```python
from build123d import *

# Parameters (mm, degrees)
F1_DEPTH = 70
F2_R     = 5
F3_R     = 2


with BuildPart() as f1:
    # F0 (on Front) → F1 (new body)
    with BuildSketch(Plane.XZ):
        Polygon((14.728606, 17.047576), (0, 17.047576), (-14.728606, 17.047576), (-5.480258, -11.053172), (0, -11.053172), (5.480258, -11.053172), align=None)
        Polygon((-7.819207, 12.047576), (0, 12.047576), (7.819207, 12.047576), (1.861998, -6.053172), (0, -6.053172), (-1.861998, -6.053172), align=None, mode=Mode.SUBTRACT)
    extrude(amount=F1_DEPTH)

    # F2
    f2_edges = [f1.edges().sort_by_distance(p)[0] for p in [
        (14.728606, -35, 17.047576),
        (5.480258, -35, -11.053172),
        (-5.480258, -35, -11.053172),
        (-14.728606, -35, 17.047576),
    ]]
    fillet(f2_edges, radius=F2_R)

    # F3
    f3_edges = [f1.edges().sort_by_distance(p)[0] for p in [
        (-1.861998, -35, -6.053172),
        (1.861998, -35, -6.053172),
        (7.819207, -35, 12.047576),
        (-7.819207, -35, 12.047576),
    ]]
    fillet(f3_edges, radius=F3_R)


solid = f1.part
```
Read the model definition and answer for the solid it produces. Units are mm, in the model's axes. A direction names the side the tool comes from. Coordinates: 2 decimals unless noted, no trailing zeros. Write each loop counter-clockwise with the first axis right and the second up, starting at its lowest first coordinate (ties: lowest second). Pieces come first, ordered by that corner, then holes. Notation, with made-up numbers: (9.25, 11) -> (39.25, 11) arc R25 ccw to (39.25, 40) -> close; hole circle Ø10 at (39.5, 88.5). An arc over 180 degrees is marked (long way). Return JSON: item names as keys, results as strings.
1. A cutting plane is placed at B-B (y = -61.5). Determine the outline of the cut face in (x, z).
Found:
{"outline": "(-12.57, 10.48) -> (-6.61, -7.62) arc R5 ccw to (-1.86, -11.05) -> (1.86, -11.05) arc R5 ccw to (6.61, -7.62) -> (12.57, 10.48) arc R5 ccw to (7.82, 17.05) -> (-7.82, 17.05) arc R5 ccw to start; hole (-6.96, 9.42) -> (-2.31, -4.68) arc R2 ccw to (-0.41, -6.05) -> (0.41, -6.05) arc R2 ccw to (2.31, -4.68) -> (6.96, 9.42) arc R2 ccw to (5.06, 12.05) -> (-5.06, 12.05) arc R2 ccw to start"}
2. A cutting plane is placed at A-A (x = -3.75). Determine the outline of the cut face in (y, z).
Found:
{"outline": "(-70, -10.68) -> (0, -10.68) -> (0, -0.32) -> (-70, -0.32) -> close; (-70, 12.05) -> (0, 12.05) -> (0, 17.05) -> (-70, 17.05) -> close"}
3. A cutting plane is placed at D-D (x = 11). Determine the outline of the cut face in (y, z).
Found:
{"outline": "(-70, 5.72) -> (0, 5.72) -> (0, 15.91) -> (-70, 15.91) -> close"}
4. A tool of negligible diameter and unlimited length cuts with its end or side. For faces 4 (the face through (0, -35, 17.048)), 5 (the face through (4.667, -34.51, 2.471)), from which of +Z, -Z, +X, -X, +Y, -Y can it reach the whole face along a straight path? Write none if from no direction.
Found:
{"face 4": "+Z, +X, -X, +Y, -Y", "face 5": "+Y, -Y"}
5. This flat-tipped pin is pushed along its axis until it touches: P1, Ø10, axis at y = -10.5, z = -4.5, coming from the -X side. Where does it stop, or does it pass through?
Found:
{"P1": "x = -9.28"}
6. Determine the mould class of faces 1 (the face through (6, 0, 3)), 2 (the face through (1.601, -35.49, -5.663)), 3 (the face through (11.83, -35.49, 15.03)) for opening direction X: pulls with the +X half, pulls with the -X half, needs draft (parallel to the pull), parting line crosses it, or undercut.
Found:
{"face 1": "needs draft", "face 2": "undercut", "face 3": "pulls with the +X half"}
7. A cutting plane is placed at C-C (z = 6.5). Determine the outline of the cut face in (x, y).
Found:
{"outline": "(-11.26, -70) -> (-5.99, -70) -> (-5.99, 0) -> (-11.26, 0) -> close; (5.99, -70) -> (11.26, -70) -> (11.26, 0) -> (5.99, 0) -> close"}
8. Find the intervals of material crossed by line 1 along Z through (x, y) = (0, -59); line 2 along X through (y, z) = (-11.5, 3); line 3 along X through (y, z) = (-16.5, -2.5), in increasing order. Write a range as from..to.
Found:
{"line 1": "-11.05..-6.05, 12.05..17.05", "line 2": "-10.11..-4.84, 4.84..10.11", "line 3": "-8.3..-3.03, 3.03..8.3"}
